Part print with two shaded views. Sizes in mm from the minimum x, y, z corner. A direction names the side the tool comes from. Coordinates: 2 decimals unless noted, no trailing zeros. Loops run counter-clockwise (first coordinate to the right, second up) from the corner with the lowest first, then second, coordinate; pieces in that order, holes last. Notation, with made-up numbers: (18.5, -22.5) -> (35.5, -22.5) arc R17 cw to (35.5, -17.5) -> close; hole circle Ø5 at (72, 2). An arc over 180 degrees is marked (long way). One line per item, written item: value. Start each with the question number.
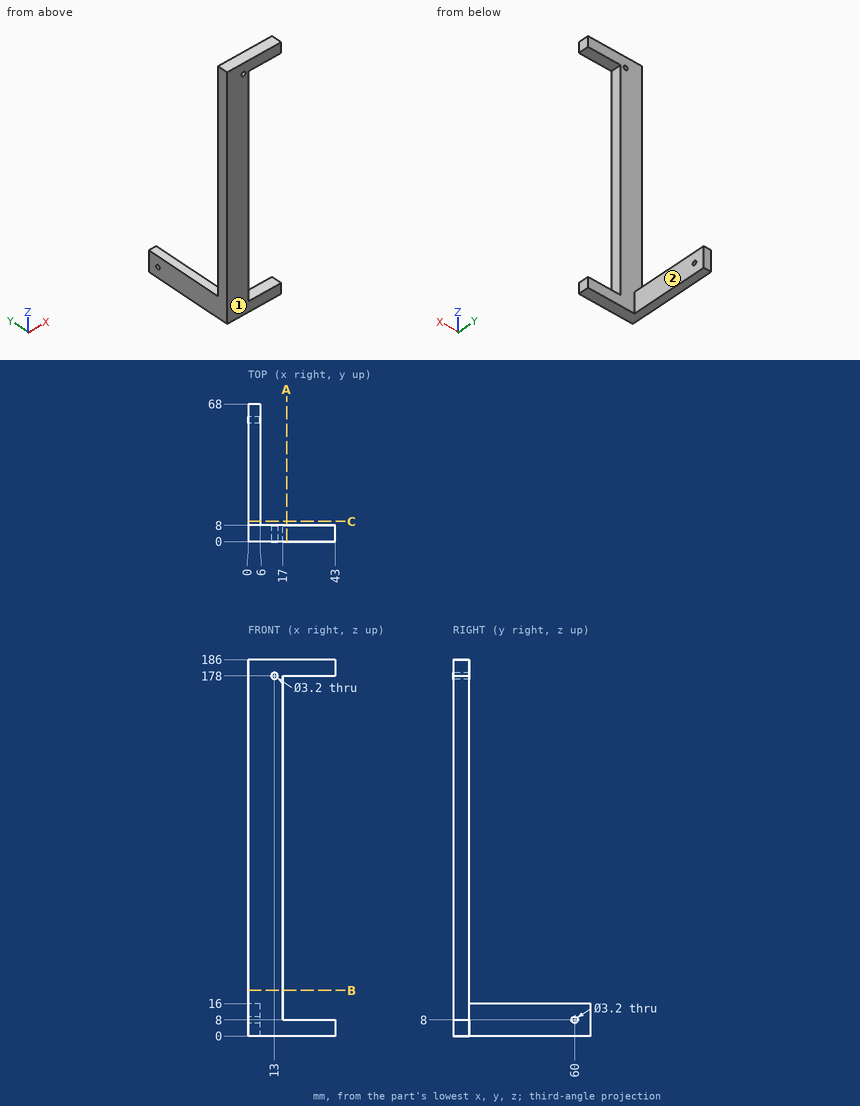
Item 1: Band-saw the part on B-B, the plane z = 22.5. List the corners of the cut face in (x, y), and give its area (3 significant figures).
Item 2: Drop flat-ended pins along their axis: pin 1 Ø3.5 at (y, z) = (60, 8) entering from +X; pin 2 Ø21.5 at (x, z) = (11, 126.5) entering from +Y; pin 3 Ø6.5 at (x, y) = (2.5, 27.5) entering from +Z. Give the stop position or say it passes through.
Item 3: Probe probe 1 along Z at (x, y) = (3.9, 60); probe 2 along Y at (x, z) = (4.7, 8); probe 3 along Y at (x, z) = (9, 102.5). List the from-to ranges inside material, lowest first.
Item 4: Band-saw the part on C-C, the plane y = 10. List the corners of the cut face in (x, z), and give its area (3 significant figures).
Item 5: Band-saw the part on A-A, the plane x = 19. List the corners of the cut face in (y, z).
Item 6: Tool access for the marked faces 1 and 2: list every direction of +Z, -Z, +X, -X, +Y, -Y with a clear straight run to the whole face (end or side of a thin tool).
Worked out:
1. outline: (0, 0) -> (17, 0) -> (17, 8) -> (0, 8) -> close
1. area: 136 mm²
2. pin 1: stops at x = 6
2. pin 2: stops at y = 8
2. pin 3: stops at z = 16
3. probe 1: z = 0 to 6.4, 9.6 to 16
3. probe 2: y = 0 to 58.4, 61.6 to 68
3. probe 3: y = 0 to 8
4. outline: (0, 0) -> (6, 0) -> (6, 16) -> (0, 16) -> close
4. area: 96.0 mm²
5. outline: (0, 0) -> (8, 0) -> (8, 8) -> (0, 8) -> close; (0, 178) -> (8, 178) -> (8, 186) -> (0, 186) -> close
6. face 1: +Z, -Z, +X, -X, -Y
6. face 2: +Z, -Z, +X, +Y
